Source: CAD feature listing. Evaluate the final solid. Frame: model axes, mm. Face numbers are marked on the shaded views. Coordinates: 2 decimals unless noted, no trailing zeros. Order: outer loops, then holes, each group sorted by start corner. A loop starts at its lowest first (then second) coordinate and runs counter-clockwise, first axis right, second up.
Item 1: Section B-B on y = 5.75. Return the cut outline in (x, z).
Item 2: Section C-C on x = 5.45. Return the cut outline in (y, z).
Item 3: Mould query, pull axis X, two halves, no side actions, for the marked faces 1 and 2. Classes: released by +X, released by -X, zero draft, split by the parting line, or undercut.
Item 4: Section A-A on x = 3.05. Return the cut outline in (y, z), then the cut area to 3 significant figures.
Item 5: Section D-D on y = 1.25. Return the cut outline in (x, z), then the cut area to 3 significant figures.
Item 6: Ray query, line 1 (Y direction, x = 3.3, z = 0.45); line 2 (Y direction, x = 1.8, z = 0.45) (3 decimals); line 3 (Z direction, x = 5.65, y = 7.5). Return the intervals inside material, ascending.
from build123d import *

# Parameters (mm, degrees)
ESQUISSE1_W        = 5.9
ESQUISSE1_H        = 8.9
BOSS_EXTRU_1_DEPTH = 0.3
BOSS_EXTRU_2_DEPTH = 0.2


with BuildPart() as part:
    # Esquisse1 → Boss.-Extru.1 (new body)
    with BuildSketch(Plane.XY):
        with Locations((2.95, 4.45)):
            Rectangle(ESQUISSE1_W, ESQUISSE1_H)
    extrude(amount=BOSS_EXTRU_1_DEPTH)

    # Esquisse2 → Boss.-Extru.2 (add)
    with BuildSketch(Plane.XY.offset(0.3)):
        Polygon((4.101145441, 4.984687707), (4.446134619, 4.632826235), (4.101145441, 4.280964763), (1.902011242, 4.280964763), (1.557022065, 4.632826235), (1.902011242, 4.984687707), align=None)
        with BuildLine():
            Line((4.628937649, 4.588843551), (4.804868385, 4.417036191))
            Line((4.804868385, 4.417036191), (4.804868385, 1.997988572))
            add(Edge.make_bspline(
                [(4.804868385, 1.997988572), (4.796892021, 1.970242627), (4.781374023, 1.916262949), (4.746481224, 1.841368841), (4.703676592, 1.774599957), (4.652323935, 1.71605919), (4.592034601, 1.666365589), (4.524746962, 1.623048736), (4.447730355, 1.590283039), (4.393174294, 1.574531191), (4.365041545, 1.566408486)],
                knots=[0, 0, 0, 0, 8.6504e-05, 0.000168293, 0.000246829, 0.000323762, 0.000400842, 0.000480537, 0.000563016, 0.000650831, 0.000650831, 0.000650831, 0.000650831], degree=3))
            Line((4.365041545, 1.566408486), (4.101145441, 2.2577613))
            Line((4.101145441, 2.2577613), (4.101145441, 4.070672555))
            Line((4.101145441, 4.070672555), (4.628937649, 4.588843551))
        make_face()
        with BuildLine():
            Line((4.189110809, 1.554038356), (1.642238515, 1.554038356))
            add(Edge.make_bspline(
                [(1.642238515, 1.554038356), (1.614492569, 1.56201472), (1.560512892, 1.577532718), (1.485618783, 1.612425517), (1.4188499, 1.655230149), (1.360309132, 1.706582806), (1.310615531, 1.76687214), (1.267298679, 1.834159779), (1.234532982, 1.911176386), (1.218781133, 1.965732447), (1.210658428, 1.993865196)],
                knots=[0, 0, 0, 0, 8.6504e-05, 0.000168293, 0.000246829, 0.000323762, 0.000400842, 0.000480537, 0.000563016, 0.000650831, 0.000650831, 0.000650831, 0.000650831], degree=3))
            Line((1.210658428, 1.993865196), (1.902011242, 2.2577613))
            Line((1.902011242, 2.2577613), (3.934835917, 2.2577613))
            Line((3.934835917, 2.2577613), (4.189110809, 1.554038356))
        make_face()
        Polygon((1.198288298, 2.169795932), (1.198288298, 4.415661733), (1.374219034, 4.587469092), (1.902011242, 4.069298096), (1.902011242, 2.4281942), align=None)
        with BuildLine():
            Line((3.933461459, 7.095856538), (1.902011242, 7.095856538))
            Line((1.902011242, 7.095856538), (1.198288298, 7.359752642))
            add(Edge.make_bspline(
                [(1.198288298, 7.359752642), (1.205668701, 7.388002372), (1.220059896, 7.443087095), (1.255578594, 7.51864428), (1.296545483, 7.587210071), (1.346696322, 7.646951249), (1.40505091, 7.698450215), (1.471609716, 7.740797307), (1.545693252, 7.776412742), (1.599339408, 7.79167572), (1.627119467, 7.799579482)],
                knots=[0, 0, 0, 0, 8.7416e-05, 0.000170454, 0.000249423, 0.000326503, 0.000403436, 0.000481973, 0.000562516, 0.00064902, 0.00064902, 0.00064902, 0.00064902], degree=3))
            Line((1.627119467, 7.799579482), (4.189110809, 7.799579482))
            Line((4.189110809, 7.799579482), (3.933461459, 7.095856538))
        make_face()
        Polygon((1.902011242, 6.925423637), (1.902011242, 5.284319741), (1.374219034, 4.766148746), (1.198288298, 4.939330564), (1.198288298, 7.183821906), align=None)
        with BuildLine():
            Line((4.101145441, 5.281570824), (4.101145441, 7.095856538))
            Line((4.101145441, 7.095856538), (4.365041545, 7.785834893))
            add(Edge.make_bspline(
                [(4.365041545, 7.785834893), (4.393174294, 7.777712188), (4.447730355, 7.761960339), (4.524746962, 7.729194642), (4.592034601, 7.68587779), (4.652323935, 7.636184189), (4.703676592, 7.577643421), (4.746481224, 7.510874538), (4.781374023, 7.435980429), (4.796892021, 7.382000752), (4.804868385, 7.354254806)],
                knots=[0, 0, 0, 0, 8.7815e-05, 0.000170294, 0.000249989, 0.000327069, 0.000404002, 0.000482539, 0.000564328, 0.000650831, 0.000650831, 0.000650831, 0.000650831], degree=3))
            Line((4.804868385, 7.354254806), (4.804868385, 4.936581646))
            Line((4.804868385, 4.936581646), (4.628937649, 4.763399828))
            Line((4.628937649, 4.763399828), (4.101145441, 5.281570824))
        make_face()
    extrude(amount=BOSS_EXTRU_2_DEPTH)


solid = part.part
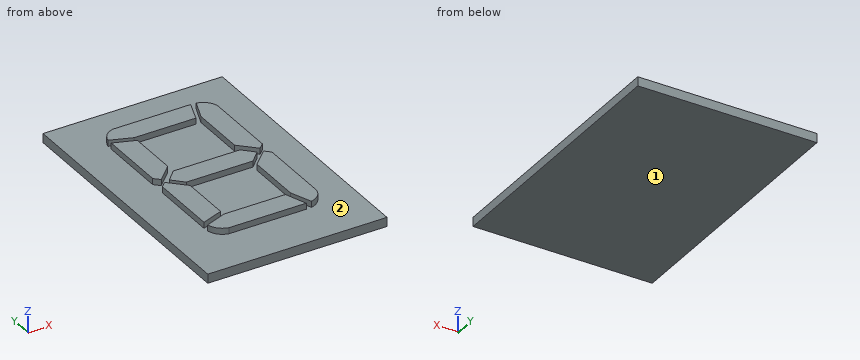
Answer list:
1. outline: (0, 0) - (5.9, 0) - (5.9, 0.3) - (4.8, 0.3) - (4.8, 0.5) - (4.1, 0.5) - (4.1, 0.3) - (1.9, 0.3) - (1.9, 0.5) - (1.2, 0.5) - (1.2, 0.3) - (0, 0.3) - close
2. outline: (0, 0) - (8.9, 0) - (8.9, 0.3) - (0, 0.3) - close
3. face 1: zero draft
3. face 2: undercut
4. outline: (0, 0) - (8.9, 0) - (8.9, 0.3) - (7.8, 0.3) - (7.8, 0.5) - (7.1, 0.5) - (7.1, 0.3) - (4.98, 0.3) - (4.98, 0.5) - (4.28, 0.5) - (4.28, 0.3) - (2.26, 0.3) - (2.26, 0.5) - (1.55, 0.5) - (1.55, 0.3) - (0, 0.3) - close
4. area: 3.09 mm2
5. outline: (0, 0) - (5.9, 0) - (5.9, 0.3) - (0, 0.3) - close
5. area: 1.77 mm2
6. line 1: y = 1.55 to 2.26, 4.28 to 4.98, 7.1 to 7.8
6. line 2: y = 1.554 to 2.219, 2.391 to 4.169, 4.385 to 4.881, 5.184 to 6.963, 7.134 to 7.8
6. line 3: z = 0 to 0.3
